The model under review builds one solid part; all positions refer to its coordinate system, in mm. A direction names the side the tool comes from. Coordinates: 2 decimals unless noted, no trailing zeros. Order: outer loops, then holes, each group sorted by start corner. A loop starts at its lowest first (then second) coordinate and runs counter-clockwise, first axis right, second up. Notation, with made-up numbers: (10, 25.25) -> (25, 25.25) arc R18 ccw to (25, 45.25) -> close; hole circle Ø10 at (-24.5, -5.75). An arc over 180 degrees is marked (long way). Answer as CSV lines item,"result". Start each with the question number.
from build123d import *
from OCP.BRepFilletAPI import BRepFilletAPI_MakeChamfer

# Parameters (mm, degrees)
BOSS_EXTRUDE1_DEPTH            = 16
SKETCH17_R                     = 5
BOSS_EXTRUDE2_DEPTH            = 6
CUT_EXTRUDE7_REACH             = 80.594
SKETCH14_R                     = 3.5
SKETCH16_W                     = 80
SKETCH16_H                     = 10
CUT_EXTRUDE8_DEPTH             = 9.5
CHAMFER3_SIZE                  = 3
CHAMFER3_SIZE_2                = 6
CBORE_FOR_M3_SHCS1_D           = 3.2
CBORE_FOR_M3_SHCS1_CBORE_D     = 5.6
CBORE_FOR_M3_SHCS1_CBORE_DEPTH = 4
CHAMFER4_SIZE                  = 10
CHAMFER4_SIZE_2                = 16.00334529
F_5_0MM_DOWEL_HOLE1_D          = 5
F_5_0MM_DOWEL_HOLE1_DEPTH      = 19
F_4_0MM_DOWEL_HOLE1_D          = 4
F_5_0MM_DOWEL_HOLE2_D          = 5
FILLET2_R                      = 5
CUT_EXTRUDE9_DEPTH             = 6
FILLET3_R                      = 4
SKETCH13_R                     = 11.5
CUT_EXTRUDE6_DEPTH             = 3
CUT_EXTRUDE10_DEPTH            = 8
FILLET4_R                      = 2


# Some blends are built 0.0001 mm under size
with BuildPart() as part:
    # Sketch1 → Boss-Extrude1 (new body)
    with BuildSketch(Plane(origin=(0, 0, 0), x_dir=(1, 0, 0), z_dir=(0, 1, 0))):
        with BuildLine():
            Line((-35, 62), (35, 62))
            ThreePointArc((35, 62), (40.656854249, 59.656854249), (43, 54))
            Line((43, 54), (43, -54))
            ThreePointArc((43, -54), (40.656854249, -59.656854249), (35, -62))
            Line((35, -62), (-35, -62))
            ThreePointArc((-35, -62), (-40.656854249, -59.656854249), (-43, -54))
            Line((-43, -54), (-43, 54))
            ThreePointArc((-43, 54), (-40.656854249, 59.656854249), (-35, 62))
        make_face()
    extrude(amount=BOSS_EXTRUDE1_DEPTH)

    # Sketch17 → Boss-Extrude2 (add)
    with BuildSketch(Plane(origin=(0, 0, 0), x_dir=(-1, 0, 0), z_dir=(0, -1, 0))):
        with Locations(Location((35, 26.5, 0), (0, 0, 270))):
            Circle(SKETCH17_R)
        with Locations(Location((-35, 26.5, 0), (0, 0, 270))):
            Circle(SKETCH17_R)
        with BuildLine():
            Line((-35, -49), (35, -49))
            ThreePointArc((35, -49), (40, -54), (35, -59))
            Line((35, -59), (-35, -59))
            ThreePointArc((-35, -59), (-40, -54), (-35, -49))
        make_face()
    extrude(amount=BOSS_EXTRUDE2_DEPTH)

    # Sketch14 → Cut-Extrude7 (cut, up to next)
    with BuildSketch(Plane(origin=(0, 16, 0), x_dir=(1, 0, 0), z_dir=(0, 1, 0)), mode=Mode.PRIVATE) as cut_extrude7_sk1:
        with Locations(Location((0, 39.569999996, 0), (0, 0, 270))):
            Circle(SKETCH14_R)
    cut_extrude7_tool1 = extrude(cut_extrude7_sk1.sketch, amount=-CUT_EXTRUDE7_REACH, mode=Mode.PRIVATE) & part.part
    add(cut_extrude7_tool1.solids().sort_by_distance((0, 16, -39.57))[0], mode=Mode.SUBTRACT)

    # Sketch16 → Cut-Extrude8 (cut)
    with BuildSketch(Plane(origin=(0, 0, 0), x_dir=(-1, 0, 0), z_dir=(0, -1, 0))):
        with Locations((0, -13.82)):
            Rectangle(SKETCH16_W, SKETCH16_H)
    extrude(amount=-CUT_EXTRUDE8_DEPTH, mode=Mode.SUBTRACT)

    # Chamfer3
    chamfer3_edges_1 = [part.edges().sort_by_distance(p)[0] for p in [
        (40, 0, 54),
    ]]
    chamfer3_side_1 = [part.faces().sort_by_distance(p)[0] for p in [
        (40.06, 0, 54),
    ]]
    chamfer3_edges_2 = [part.edges().sort_by_distance(p)[0] for p in [
        (0, 0, 59),
    ]]
    chamfer3_side_2 = [part.faces().sort_by_distance(p)[0] for p in [
        (0, 0, 59.06),
    ]]
    chamfer3_edges_3 = [part.edges().sort_by_distance(p)[0] for p in [
        (0, 0, 49),
    ]]
    chamfer3_side_3 = [part.faces().sort_by_distance(p)[0] for p in [
        (0, 0, 48.94),
    ]]
    chamfer3_edges_4 = [part.edges().sort_by_distance(p)[0] for p in [
        (-40, 0, 54),
    ]]
    chamfer3_side_4 = [part.faces().sort_by_distance(p)[0] for p in [
        (-40.06, 0, 54),
    ]]
    chamfer3_edges_5 = [part.edges().sort_by_distance(p)[0] for p in [
        (-35, 0, -31.5),
    ]]
    chamfer3_side_5 = [part.faces().sort_by_distance(p)[0] for p in [
        (-35, 0, -31.56),
    ]]
    chamfer3_edges_6 = [part.edges().sort_by_distance(p)[0] for p in [
        (35, 0, -31.5),
    ]]
    chamfer3_side_6 = [part.faces().sort_by_distance(p)[0] for p in [
        (35, 0, -31.56),
    ]]
    chamfer3 = BRepFilletAPI_MakeChamfer(part.part.solid().wrapped)
    for e in chamfer3_edges_1:
        chamfer3.Add(CHAMFER3_SIZE - 0.0001, CHAMFER3_SIZE_2 - 0.0001, e.wrapped, chamfer3_side_1[0].wrapped)
    for e in chamfer3_edges_2:
        chamfer3.Add(CHAMFER3_SIZE - 0.0001, CHAMFER3_SIZE_2 - 0.0001, e.wrapped, chamfer3_side_2[0].wrapped)
    for e in chamfer3_edges_3:
        chamfer3.Add(CHAMFER3_SIZE - 0.0001, CHAMFER3_SIZE_2 - 0.0001, e.wrapped, chamfer3_side_3[0].wrapped)
    for e in chamfer3_edges_4:
        chamfer3.Add(CHAMFER3_SIZE - 0.0001, CHAMFER3_SIZE_2 - 0.0001, e.wrapped, chamfer3_side_4[0].wrapped)
    for e in chamfer3_edges_5:
        chamfer3.Add(CHAMFER3_SIZE - 0.0001, CHAMFER3_SIZE_2 - 0.0001, e.wrapped, chamfer3_side_5[0].wrapped)
    for e in chamfer3_edges_6:
        chamfer3.Add(CHAMFER3_SIZE - 0.0001, CHAMFER3_SIZE_2 - 0.0001, e.wrapped, chamfer3_side_6[0].wrapped)
    add(Compound.cast(chamfer3.Shape()), mode=Mode.REPLACE)  # a hair under: the kernel refuses the full size

    # CBORE for M3 SHCS1 (through all)
    with Locations(Plane(origin=(0, 16, 0), x_dir=(1, 0, 0), z_dir=(0, 1, 0))):
        with Locations((-15.5, 55.069999996), (-15.5, 24.069999996), (15.5, 24.069999996), (15.5, 55.069999996)):
            CounterBoreHole(CBORE_FOR_M3_SHCS1_D / 2, CBORE_FOR_M3_SHCS1_CBORE_D / 2, CBORE_FOR_M3_SHCS1_CBORE_DEPTH)

    # Chamfer4
    # the kernel refuses this chamfer: 16.00334529, 10 mm, written as the material it adds along each edge
    with BuildSketch(Plane(origin=(40, 9.5, -32.554216019), x_dir=(0.05243311939005598, -0.9986244379099823, 0), z_dir=(0, 0, 1))) as chamfer4_piece_1_section:
        Polygon((CHAMFER4_SIZE * 0.99862443791, -CHAMFER4_SIZE * 0.0524331193901), (-CHAMFER4_SIZE_2 * 0.0524331193914, -CHAMFER4_SIZE_2 * 0.998624437936), (0, 0), align=None)
    chamfer4_piece_1 = extrude(amount=92.748432037, mode=Mode.PRIVATE)
    chamfer4_piece_1 = split(chamfer4_piece_1, bisect_by=Plane(origin=(34.599202333, 0, -11.867108009), z_dir=(0, 1, 0)), keep=Keep.TOP, mode=Mode.PRIVATE)
    add(chamfer4_piece_1)
    with BuildSketch(Plane(origin=(-40, 9.5, 60.194216019), x_dir=(-0.05243311939005598, -0.9986244379099823, 0), z_dir=(0, 0, -1))) as chamfer4_piece_2_section:
        Polygon((CHAMFER4_SIZE * 0.99862443791, -CHAMFER4_SIZE * 0.0524331193901), (-CHAMFER4_SIZE_2 * 0.0524331193914, -CHAMFER4_SIZE_2 * 0.998624437936), (0, 0), align=None)
    chamfer4_piece_2 = extrude(amount=92.748432037, mode=Mode.PRIVATE)
    chamfer4_piece_2 = split(chamfer4_piece_2, bisect_by=Plane(origin=(-34.599202333, 0, 39.507108009), z_dir=(0, 1, 0)), keep=Keep.TOP, mode=Mode.PRIVATE)
    add(chamfer4_piece_2)

    # Ø5.0mm Dowel Hole1
    with Locations(Plane.XZ.offset(6)):
        with Locations((-35, 54), (35, 54), (-35, -26.5), (35, -26.5)):
            Hole(F_5_0MM_DOWEL_HOLE1_D / 2, depth=F_5_0MM_DOWEL_HOLE1_DEPTH)

    # Ø4.0mm Dowel Hole1 (through all)
    with Locations(Plane(origin=(0, 16, 0), x_dir=(1, 0, 0), z_dir=(0, 1, 0))):
        with Locations((0, -13.82)):
            Hole(F_4_0MM_DOWEL_HOLE1_D / 2)

    # Ø5.0mm Dowel Hole2 (through all)
    with Locations(Plane(origin=(0, 16, 0), x_dir=(1, 0, 0), z_dir=(0, 1, 0))):
        with Locations((0, -22.680000004)):
            Hole(F_5_0MM_DOWEL_HOLE2_D / 2)

    # Fillet2
    fillet2_edges = [part.edges().sort_by_distance(p)[0] for p in [
        (39.199832735, 0, 13.82),
        (-39.199832735, 0, 13.82),
    ]]
    fillet(fillet2_edges, radius=FILLET2_R)

    # Sketch26 → Cut-Extrude9 (cut)
    with BuildSketch(Plane.XZ):
        Polygon((22.15, -80.719999996), (-22.15, -80.719999996), (-22.15, -22.005786434), (-17.564213562, -17.419999996), (17.564213562, -17.419999996), (22.15, -22.005786434), align=None)
    extrude(amount=-CUT_EXTRUDE9_DEPTH, mode=Mode.SUBTRACT)

    # Fillet3
    fillet3_edges = [part.edges().sort_by_distance(p)[0] for p in [
        (-22.15, 3, -62),
        (22.15, 3, -62),
    ]]
    fillet(fillet3_edges, radius=FILLET3_R)

    # Sketch13 → Cut-Extrude6 (cut)
    with BuildSketch(Plane.XZ.offset(-6)):
        with Locations(Location((0, -39.569999996, 0), (0, 0, 270))):
            Circle(SKETCH13_R)
    extrude(amount=-CUT_EXTRUDE6_DEPTH, mode=Mode.SUBTRACT)

    # Sketch28 → Cut-Extrude10 (cut)
    with BuildSketch(Plane(origin=(0, 0, 0), x_dir=(-1, 0, 0), z_dir=(0, -1, 0))):
        Polygon((4.965212315, -22.680000004), (2.482606157, -18.380000004), (-2.482606158, -18.380000004), (-4.965212315, -22.680000004), (-2.482606158, -26.980000004), (2.482606157, -26.980000004), align=None)
    extrude(amount=-CUT_EXTRUDE10_DEPTH, mode=Mode.SUBTRACT)

    # Fillet4
    fillet4_edges = [part.edges().sort_by_distance(p)[0] for p in [
        (-3.850926294, 0, 20.750000002),
        (3.850926295, 0, 20.750000002),
        (3.723909237, 0, 24.830000004),
        (0, 0, 26.980000004),
        (-3.723909236, 0, 24.830000004),
    ]]
    fillet(fillet4_edges, radius=FILLET4_R)


solid = part.part
1) Consider section B-B (y = -3.75). Give the boundary of the cut face in (x, z).
2) Wall thickness on L1, parallel to Z at x = 15.5, y = 10.55; L2, parallel to Z at x = 15.5, y = 14.8; L3, parallel to X at y = 4.5, z = -45.5: over which ranges is each line inside the solid? List them lowest first. Write a range as [from, to].
3) Mouldability with a two-part tool opening along Z and no side actions: class faces 4 (the face through (-14.23, 8.96, -23.1)), 5 (the face through (12, 6, -39)), 6 (the face through (-40.719, 7.888, -59.594)) as released by +Z, released by -Z, zero draft, split by the parting line, or undercut.
4) Tool access review of faces 1 (the face through (-14, 12, -23)), 2 (the face through (4.22, 0.57, 25.17)), 3 (the face through (-23.353, 2.958, -60.859)): name each direction out of +Z, -Z, +X, -X, +Y, -Y from which nothing blocks a thin tool from reaching the whole face with its end or side.
5) Consider section C-C (z = 0.5). Give the boundary of the cut face in (x, y), plus the area to 3 significant figures.
6) Consider section A-A (z = -39.57). Give the boundary of the cut face in (x, y), plus the area to 3 significant figures.
7) Insertion check: pin 1 Ø7.5 at (x, z) = (-15.5, -24.07) entering from -Y; pin 2 Ø8 at (x, y) = (-2.5, -3.5) entering from -Z; pin 3 Ø3 at (x, z) = (16, -55.5) entering from +Y. Each pin has a flat end and moves straight along its axis. Give the tip position at first contact, or say it passes through.
Result:
1,outline,"circle Ø12.25 at (-35, -26.5); (-35, 47.88) -> (35, 47.88) arc R6.12 ccw to (35, 60.12) -> (-35, 60.12) arc R6.12 ccw to start; circle Ø12.25 at (35, -26.5); hole circle Ø5 at (-35, -26.5); hole circle Ø5 at (-35, 54); hole circle Ø5 at (35, -26.5); hole circle Ø5 at (35, 54)"
2,L1,"[-62, -56.67], [-53.47, -25.67], [-22.47, 62]"
2,L2,"[-62, -57.87], [-52.27, -26.87], [-21.27, 62]"
2,L3,"[-43, -22.15], [22.15, 43]"
3,face 4,"undercut"
3,face 5,"zero draft"
3,face 6,"released by -Z"
4,face 1,"+Y"
4,face 2,"-Y"
4,face 3,"-Z, -Y"
5,outline,"(-43, 0) -> (43, 0) -> (43, 16) -> (-43, 16) -> close"
5,area,"1,380 mm2"
6,outline,"(-43, 0) -> (-22.15, 0) -> (-22.15, 6) -> (-11.5, 6) -> (-11.5, 9) -> (-3.5, 9) -> (-3.5, 16) -> (-43, 16) -> close; (3.5, 9) -> (11.5, 9) -> (11.5, 6) -> (22.15, 6) -> (22.15, 0) -> (43, 0) -> (43, 16) -> (3.5, 16) -> close"
6,area,"992 mm2"
7,pin 1,"y = 6"
7,pin 2,"z = -17.42"
7,pin 3,"y = 12"
